Here's the drawing with two shaded views (mm, measured from the low corner). I have some questions. Round coordinates to 2 decimals unless told otherwise and drop trailing zeros. Write each loop counter-clockwise with the first axis right and the second up, starting at its lowest first coordinate (ties: lowest second). Pieces come first, ordered by that corner, then holes. Notation, with made-up numbers: M 43,77 L 70,77 A18 ccw 70,105 Z; hole C -20,-20.75 d4. An arc over 180 degrees is marked long. Write item = value, one per line. Start each with the question number.
(1) I want a section at B-B (x = 19.05). List the corners of the cut face in (y, z) for me (3 decimals).
(2) I want a section at A-A (z = 19.05). List the corners of the cut face in (x, y) for me (3 decimals).
(3) Will these pins go through, and if not, where does the flat tip stop? pin 1 Ø4 at (y, z) = (11, 11) entering from -X; pin 2 Ø5 at (y, z) = (5.5, 6) entering from -X; pin 3 Ø3 at (x, z) = (14.5, 28) entering from -Y (1 decimal); pin 4 Ø6 at (x, y) = (34, 1.5) entering from +Z.
(4) I want a section at D-D (y = 11.25). List the corners of the cut face in (x, z) for me (3 decimals).
(5) I need wall thicknesses on line 1 along Z through (x, y) = (19.05, 5.25) (3 decimals); line 2 along Y through (x, z) = (4, 19); line 3 along Z through (x, y) = (36, 6.35) (3 decimals). Which ranges of each line are inside material? Lowest first, please.
(6) I want a section at C-C (y = 6.25). List the corners of the cut face in (x, z) for me (3 decimals), and give its area (3 significant figures).
(7) If we mould it in two halves opening along Y, with no side actions, what happens to the marked faces 1, 2 and 3? For each: released by +Y, released by -Y, zero draft, split by the parting line, or undercut.
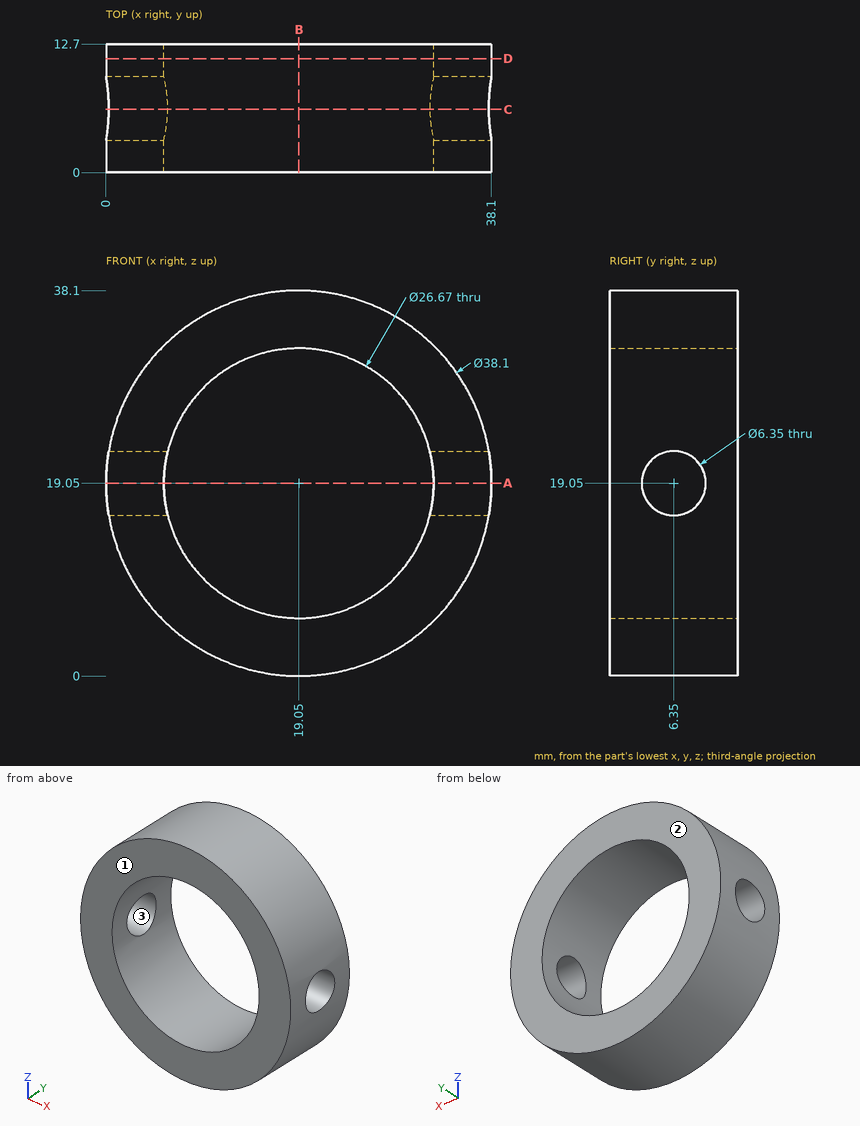
Returned:
q1.outline = M 0,0 L 12.7,0 L 12.7,5.715 L 0,5.715 Z; M 0,32.385 L 12.7,32.385 L 12.7,38.1 L 0,38.1 Z
q2.outline = M 0,0 L 5.715,0 L 5.715,3.175 L 0,3.175 Z; M 0,9.525 L 5.715,9.525 L 5.715,12.7 L 0,12.7 Z; M 32.385,0 L 38.1,0 L 38.1,3.175 L 32.385,3.175 Z; M 32.385,9.525 L 38.1,9.525 L 38.1,12.7 L 32.385,12.7 Z
q3.pin_1 = 0.99
q3.pin_2 = 3.19
q3.pin_3 = through
q3.pin_4 = 33.89
q4.outline = C 19.05,19.05 d38.1; hole C 19.05,19.05 d26.67
q5.line_1 = 0 to 5.715, 32.385 to 38.1
q5.line_2 = 0 to 3.18, 9.52 to 12.7
q5.line_3 = 10.355 to 15.875, 22.225 to 27.745
q6.outline = M 0.266,15.877 A19.05 ccw 37.834,15.877 L 32.002,15.877 A13.335 cw 6.098,15.877 Z; M 0.266,22.223 L 6.098,22.223 A13.335 cw 32.002,22.223 L 37.834,22.223 A19.05 ccw Z
q6.area = 508 mm²
q7.face_1 = released by -Y
q7.face_2 = released by +Y
q7.face_3 = undercut
